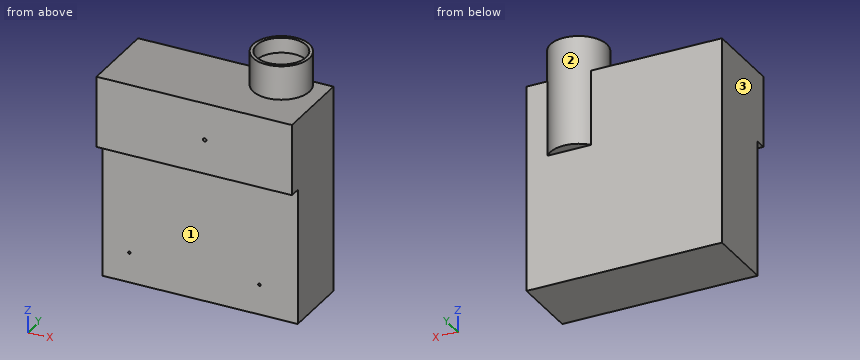
```python
from build123d import *

# Parameters (mm, degrees)
SKETCH_1_W             = 260
SKETCH_1_H             = 275
EXTRUDE_1_DEPTH        = 107
EXTRUDE_2_DEPTH        = 25
EXTRUDE_2_DEPTH_BACK   = 100
SKETCH_2_R             = 37.5
SKETCH_3_W             = 180.515861549
SKETCH_3_H             = 15
CUT_EXTRUDE_1_DEPTH    = 398.171562426
M4X0_7_1_D             = 3.3
M4X0_7_1_DEPTH         = 11.5
M4X0_7_1_TIP           = 0.991420021
SKETCH_17_R            = 37.5
SKETCH_17_R_2          = 33.067386868
EXTRUDE_4_DEPTH        = 20
HOLE_WIZARD_M4_1_D     = 4.5
HOLE_WIZARD_M4_1_DEPTH = 20
HOLE_WIZARD_M4_1_TIP   = 1.351936393


with BuildPart() as part:
    # Sketch 1 → 보스-돌출1 (new body)
    with BuildSketch(Plane(origin=(0, 0, 0), x_dir=(1, 0, 0), z_dir=(0, 1, 0))):
        with Locations((130, 137.5)):
            Rectangle(SKETCH_1_W, SKETCH_1_H)
    extrude(amount=EXTRUDE_1_DEPTH)

    # Sketch 2 → 보스-돌출2 (add, two sides: drawn at the far end of the back side and taken through both)
    with BuildSketch(Plane.XY.offset(-EXTRUDE_2_DEPTH_BACK)):
        with Locations((203, 83)):
            Circle(SKETCH_2_R)
    extrude(amount=EXTRUDE_2_DEPTH + EXTRUDE_2_DEPTH_BACK)

    # 스케치3 → 컷-돌출1 (cut, through all)
    with BuildSketch(Plane(origin=(260, 0, 0), x_dir=(0, 0, -1), z_dir=(1, 0, 0))):
        with Locations((184.742069226, 7.5)):
            Rectangle(SKETCH_3_W, SKETCH_3_H)
    extrude(amount=-CUT_EXTRUDE_1_DEPTH, mode=Mode.SUBTRACT)

    # M4x0.7 나사 구멍1
    with Locations(Plane(origin=(0, 15, 0), x_dir=(-1, 0, 0), z_dir=(0, -1, 0))):
        with Locations((-36, 235), (-209, 235)):
            Hole(M4X0_7_1_D / 2, depth=M4X0_7_1_DEPTH)
            with Locations((0, 0, -(M4X0_7_1_DEPTH + M4X0_7_1_TIP / 2))):  # 118° drill point
                Cone(0, M4X0_7_1_D / 2, M4X0_7_1_TIP, mode=Mode.SUBTRACT)

    # 스케치17 → 보스-돌출4 (add)
    with BuildSketch(Plane.XY.offset(25)):
        with Locations((203, 83)):
            Circle(SKETCH_17_R)
        with Locations((203, 83)):
            Circle(SKETCH_17_R_2, mode=Mode.SUBTRACT)
    extrude(amount=EXTRUDE_4_DEPTH)

    # M4 여유 구멍1
    with Locations(Plane(origin=(0, 0, 0), x_dir=(-1, 0, 0), z_dir=(0, -1, 0))):
        with Locations((-143.933526012, 49.055508383)):
            Hole(HOLE_WIZARD_M4_1_D / 2, depth=HOLE_WIZARD_M4_1_DEPTH)
            with Locations((0, 0, -(HOLE_WIZARD_M4_1_DEPTH + HOLE_WIZARD_M4_1_TIP / 2))):  # 118° drill point
                Cone(0, HOLE_WIZARD_M4_1_D / 2, HOLE_WIZARD_M4_1_TIP, mode=Mode.SUBTRACT)


solid = part.part
```
Geometry check sheet. Reference: the model listing, model coordinates, mm. Face numbers are marked on the shaded views. A direction names the side the tool comes from. Coordinates: 2 decimals unless noted, no trailing zeros. Loops run counter-clockwise (first coordinate to the right, second up) from the corner with the lowest first, then second, coordinate; pieces in that order, holes last.
Item 1: Sectioned sample at D-D, the plane y = 11. Record the boundary of the cut face in (x, z), then the cut area to 4 significant figures.
Item 2: Go/stop test with flat-tipped pins: pin 1 Ø4 at (x, z) = (227, -124) entering from +Y; pin 2 Ø3 at (x, z) = (217.5, 5.5) entering from +Y; pin 3 Ø1 at (x, z) = (199.5, -68) entering from +Y. Record where each tip stops, or that it passes through.
Item 3: Sectioned sample at C-C, the plane z = 11. Record the boundary of the cut face in (x, y), then the cut area to 3 significant figures.
Item 4: Sectioned sample at B-B, the plane x = 24. Record the boundary of the cut face in (y, z).
Item 5: Thickness scan on line 1 (X direction, y = 21, z = -235); line 2 (Y direction, x = 203, z = 30.5); line 3 (Y direction, x = 139, z = -92.5). Record the ranges inside material, lowest first.
Item 6: Access from +Z, -Z, +X, -X, +Y, -Y to the whole of each face (thin tool, end or side, straight path). Record for the marked faces 1, 2 and 3.
Item 7: Sectioned sample at A-A, the plane y = 83. Record the boundary of the cut face in (x, z).
Check result:
1. outline: (0, -94.48) - (260, -94.48) - (260, 0) - (0, 0) - close; hole circle Ø4.5 at (143.93, -49.06)
1. area: 24,550 mm2
2. pin 1: stops at y = 107
2. pin 2: stops at y = 118.17
2. pin 3: stops at y = 120.38
3. outline: circle Ø75 at (203, 83)
3. area: 4,420 mm2
4. outline: (0, -94.48) - (15, -94.48) - (15, -275) - (107, -275) - (107, 0) - (0, 0) - close
5. line 1: x = 0 to 34.35, 37.65 to 207.35, 210.65 to 260
5. line 2: y = 45.5 to 49.93, 116.07 to 120.5
5. line 3: y = 0 to 107
6. face 1: -Z, +X, -X, -Y
6. face 2: +Z
6. face 3: +Z, -Z, -X, +Y, -Y
7. outline: (0, -275) - (260, -275) - (260, 0) - (240.5, 0) - (240.5, 45) - (236.07, 45) - (236.07, 25) - (169.93, 25) - (169.93, 45) - (165.5, 45) - (165.5, 0) - (0, 0) - close
